from build123d import *

# Parameters (mm, degrees)
SKETCH1_R           = 10
BOSS_EXTRUDE1_DEPTH = 8
BOSS_EXTRUDE3_DEPTH = 2
SKETCH6_R           = 3
CUT_EXTRUDE1_DEPTH  = 128.644036288


with BuildPart() as part:
    # Sketch1 → Boss-Extrude1 (new body)
    with BuildSketch(Plane(origin=(0, 0, 0), x_dir=(1, 0, 0), z_dir=(0, 1, 0))):
        with Locations(Location((0, 0, 0), (0, 0, 270))):
            Circle(SKETCH1_R)
    extrude(amount=BOSS_EXTRUDE1_DEPTH)

    # Sketch5 → Boss-Extrude3 (add)
    with BuildSketch(Plane(origin=(0, 0, 0), x_dir=(1, 0, 0), z_dir=(0, 1, 0))):
        with BuildLine():
            Line((-119, 8), (119, 8))
            ThreePointArc((119, 8), (127, 0), (119, -8))
            Line((119, -8), (-119, -8))
            ThreePointArc((-119, -8), (-127, 0), (-119, 8))
        make_face()
    extrude(amount=BOSS_EXTRUDE3_DEPTH)

    # Sketch6 → Cut-Extrude1 (cut, through all)
    with BuildSketch(Plane(origin=(0, 0, 0), x_dir=(1, 0, 0), z_dir=(0, 1, 0))):
        with Locations(Location((0, 0, 0), (0, 0, 270))):
            Circle(SKETCH6_R)
    extrude(amount=CUT_EXTRUDE1_DEPTH, mode=Mode.SUBTRACT)


solid = part.part
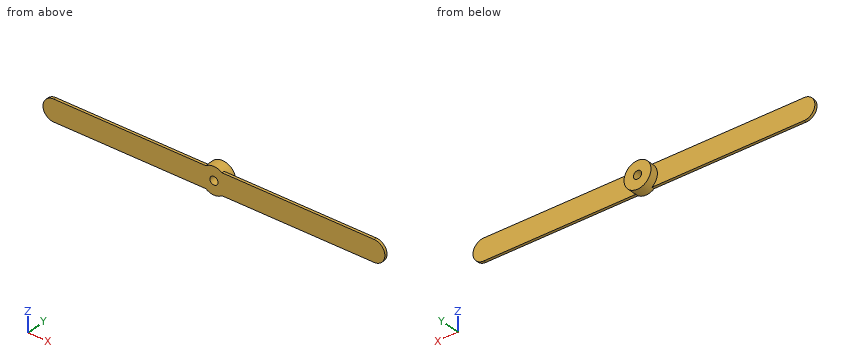
Verification items for the finished model (mm, model axes). Give positions to 0.01 mm unless a question says otherwise; leave off trailing zeros. Loops run counter-clockwise (first coordinate to the right, second up) from the corner with the lowest first, then second, coordinate; pieces in that order, holes last.
1) Depth check by flat-ended pin: pin 1 Ø1 at (y, z) = (7, 5.5) entering from +X; pin 2 Ø5 at (x, z) = (60.5, 1.5) entering from +Y; pin 3 Ø1.6 at (x, y) = (59.5, 1.5) entering from +Z. Enter the tip coordinate at first touch or a pass-through.
2) Sectioned sample at B-B, the plane x = 0. Enter the section's corners in (y, z), then the cut area to 3 significant figures.
3) Sectioned sample at C-C, the plane y = 4. Enter the section's corners in (x, z).
4) Sectioned sample at D-D, the plane x = 42. Enter the section's corners in (y, z), then the cut area to 3 significant figures.
5) Sectioned sample at A-A, the plane z = 0. Enter the section's corners in (x, y), then the cut area to 3 significant figures.
6) Thickness scan on line 1 along X through (y, z) = (4.75, 0); line 2 along Y through (x, z) = (-88.5, 3). Record the ranges inside material, lowest first.
Answers:
1. pin 1: stops at x = 8.66
1. pin 2: stops at y = 2
1. pin 3: stops at z = 8
2. outline: (0, -10) - (8, -10) - (8, -3) - (0, -3) - close; (0, 3) - (8, 3) - (8, 10) - (0, 10) - close
2. area: 112 mm2
3. outline: circle Ø20 at (0, 0); hole circle Ø6 at (0, 0)
4. outline: (0, -8) - (2, -8) - (2, 8) - (0, 8) - close
4. area: 32.0 mm2
5. outline: (-127, 0) - (-3, 0) - (-3, 8) - (-10, 8) - (-10, 2) - (-127, 2) - close; (3, 0) - (127, 0) - (127, 2) - (10, 2) - (10, 8) - (3, 8) - close
5. area: 580 mm2
6. line 1: x = -10 to -3, 3 to 10
6. line 2: y = 0 to 2
